from build123d import *

# Parameters (mm, degrees)
BASE_DEPTH                   = 12.7
BASE_DEPTH_BACK              = 12.7
SKETCH1_W                    = 43.18
SKETCH1_H                    = 108.204
ACTUATORPLANECUT_DEPTH       = 6.0325
CENTERSLOT_DEPTH             = 60.619162222
CENTERSLOT_DEPTH_BACK        = 60.619162222
SKETCH5_W                    = 25.654
SKETCH5_H                    = 19.05
SHAFTGUIDE_REACH             = 113.065
SKETCH2_R                    = 4.7625
CENTERSLOTFILLET_R           = 3.175
GEARBOXPIT_DEPTH             = 11.176
FRONTCUTAWAY_DEPTH           = 15.24
GEARBOXSLOTSH_DEPTH          = 2.286
TOGGLEASSEMHOLES_D           = 2.7051
TOGGLEASSEMHOLES_DEPTH       = 9.398
TOGGLEASSEMHOLES_TIP         = 0.81269403
GEARBOXMOUNTINGHOLES_D       = 2.7051
GEARBOXMOUNTINGHOLES_DEPTH   = 9.398
GEARBOXMOUNTINGHOLES_TIP     = 0.81269403
CAPMOUNTINGHOLES_D           = 3.6576
CAPMOUNTINGHOLES_CBORE_D     = 7.14502
CAPMOUNTINGHOLES_CBORE_DEPTH = 3.5052
ROLLMOTORSLOT_REACH          = 113.065


with BuildPart() as part:
    # Sketch1 → Base (new, two sides: drawn at the far end of the back side and taken through both)
    with BuildSketch(Plane(origin=(0, 0, 0), x_dir=(1, 0, 0), z_dir=(0, 1, 0)).offset(-BASE_DEPTH_BACK)):
        Rectangle(SKETCH1_W, SKETCH1_H)
    extrude(amount=BASE_DEPTH + BASE_DEPTH_BACK)

    # Sketch3 → ActuatorPlaneCut (cut)
    with BuildSketch(Plane(origin=(0, -12.7, 0), x_dir=(-1, 0, 0), z_dir=(0, -1, 0))):
        Polygon((10.922, -28.702), (16.256, -28.702), (21.59, -28.702), (21.59, -54.102), (-21.59, -54.102), (-21.59, -28.702), (-10.922, -28.702), (-10.922, -11.176), (10.922, -11.176), align=None)
    extrude(amount=-ACTUATORPLANECUT_DEPTH, mode=Mode.SUBTRACT)

    # Sketch5 → CenterSlot (cut, two sides: drawn at the far end of the back side and taken through both)
    with BuildSketch(Plane(origin=(0, 0, 0), x_dir=(1, 0, 0), z_dir=(0, 1, 0)).offset(-CENTERSLOT_DEPTH_BACK)):
        with Locations((0, 0.127)):
            Rectangle(SKETCH5_W, SKETCH5_H)
    extrude(amount=CENTERSLOT_DEPTH + CENTERSLOT_DEPTH_BACK, mode=Mode.SUBTRACT)

    # Sketch2 → ShaftGuide (cut, up to next)
    with BuildSketch(Plane(origin=(0, 0, -54.102), x_dir=(-1, 0, 0), z_dir=(0, 0, -1)), mode=Mode.PRIVATE) as shaftguide_sk1:
        with Locations((0, -12.7)):
            Circle(SKETCH2_R)
    shaftguide_tool1 = extrude(shaftguide_sk1.sketch, amount=-SHAFTGUIDE_REACH, mode=Mode.PRIVATE) & part.part
    add(shaftguide_tool1.solids().sort_by_distance((0, -12.7, -54.102))[0], mode=Mode.SUBTRACT)

    # CenterSlotFillet
    centerslotfillet_edges = [part.edges().sort_by_distance(p)[0] for p in [
        (-12.827, 0, -9.652),
        (-12.827, 0, 9.398),
        (12.827, 0, 9.398),
        (12.827, 0, -9.652),
    ]]
    fillet(centerslotfillet_edges, radius=CENTERSLOTFILLET_R)

    # Sketch40 → GearBoxPit (cut)
    with BuildSketch(Plane.XZ.offset(12.7)):
        with BuildLine():
            Line((10.922, 6.858), (-10.922, 6.858))
            Line((-10.922, 6.858), (-10.922, 25.527))
            ThreePointArc((-10.922, 25.527), (-9.99206403, 27.77206403), (-7.747, 28.702))
            Line((-7.747, 28.702), (7.747, 28.702))
            ThreePointArc((7.747, 28.702), (9.99206403, 27.77206403), (10.922, 25.527))
            Line((10.922, 25.527), (10.922, 6.858))
        make_face()
    extrude(amount=-GEARBOXPIT_DEPTH, mode=Mode.SUBTRACT)

    # Sketch60 → FrontCutaway (cut)
    with BuildSketch(Plane(origin=(0, 12.7, 0), x_dir=(1, 0, 0), z_dir=(0, 1, 0))):
        with BuildLine():
            Line((-12.827, 6.477), (12.827, 6.477))
            Line((12.827, 6.477), (12.827, 25.527))
            ThreePointArc((12.827, 25.527), (11.89706403, 27.77206403), (9.652, 28.702))
            Line((9.652, 28.702), (-9.652, 28.702))
            ThreePointArc((-9.652, 28.702), (-11.89706403, 27.77206403), (-12.827, 25.527))
            Line((-12.827, 25.527), (-12.827, 6.477))
        make_face()
    extrude(amount=-FRONTCUTAWAY_DEPTH, mode=Mode.SUBTRACT)

    # Sketch67 → GearBoxSlotsH (cut)
    with BuildSketch(Plane(origin=(0, -12.7, 0), x_dir=(-1, 0, 0), z_dir=(0, -1, 0))):
        with BuildLine():
            Line((-12.3825, -12.811125), (12.3825, -12.811125))
            ThreePointArc((12.3825, -12.811125), (12.779375, -13.208), (12.3825, -13.604875))
            Line((12.3825, -13.604875), (-12.3825, -13.604875))
            ThreePointArc((-12.3825, -13.604875), (-12.779375, -13.208), (-12.3825, -12.811125))
        make_face()
        with BuildLine():
            Line((-12.3825, -23.479125), (12.3825, -23.479125))
            ThreePointArc((12.3825, -23.479125), (12.779375, -23.876), (12.3825, -24.272875))
            Line((12.3825, -24.272875), (-12.3825, -24.272875))
            ThreePointArc((-12.3825, -24.272875), (-12.779375, -23.876), (-12.3825, -23.479125))
        make_face()
    extrude(amount=-GEARBOXSLOTSH_DEPTH, mode=Mode.SUBTRACT)

    # ToggleAssemHoles
    with Locations(Plane(origin=(0, -12.7, 0), x_dir=(-1, 0, 0), z_dir=(0, -1, 0))):
        with Locations((15.875, 22.352), (-15.875, 22.352)):
            Hole(TOGGLEASSEMHOLES_D / 2, depth=TOGGLEASSEMHOLES_DEPTH)
            with Locations((0, 0, -(TOGGLEASSEMHOLES_DEPTH + TOGGLEASSEMHOLES_TIP / 2))):  # 118° drill point
                Cone(0, TOGGLEASSEMHOLES_D / 2, TOGGLEASSEMHOLES_TIP, mode=Mode.SUBTRACT)

    # GearBoxMountingHoles
    with Locations(Plane(origin=(0, -12.7, 0), x_dir=(-1, 0, 0), z_dir=(0, -1, 0))):
        with Locations((-16.256, -18.542), (16.256, -18.542)):
            Hole(GEARBOXMOUNTINGHOLES_D / 2, depth=GEARBOXMOUNTINGHOLES_DEPTH)
            with Locations((0, 0, -(GEARBOXMOUNTINGHOLES_DEPTH + GEARBOXMOUNTINGHOLES_TIP / 2))):  # 118° drill point
                Cone(0, GEARBOXMOUNTINGHOLES_D / 2, GEARBOXMOUNTINGHOLES_TIP, mode=Mode.SUBTRACT)

    # CapMountingHoles (through all)
    with Locations(Plane(origin=(-0.837932951, 12.7, 8.633720573), x_dir=(-1, 0, 0), z_dir=(0, 1, 0))):
        with Locations((-13.537932951, 36.578279427), (11.862067049, 36.578279427)):
            CounterBoreHole(CAPMOUNTINGHOLES_D / 2, CAPMOUNTINGHOLES_CBORE_D / 2, CAPMOUNTINGHOLES_CBORE_DEPTH)

    # Sketch81 → RollMotorSlot (cut, up to next)
    with BuildSketch(Plane(origin=(0, 0, -54.102), x_dir=(-1, 0, 0), z_dir=(0, 0, -1)), mode=Mode.PRIVATE) as rollmotorslot_sk1:
        with BuildLine():
            Line((10.16, 12.7), (-10.16, 12.7))
            Line((-10.16, 12.7), (-10.16, 8.46582))
            ThreePointArc((-10.16, 8.46582), (-7.370192091, 1.730627909), (-0.635, -1.05918))
            Line((-0.635, -1.05918), (0.635, -1.05918))
            ThreePointArc((0.635, -1.05918), (7.370192091, 1.730627909), (10.16, 8.46582))
            Line((10.16, 8.46582), (10.16, 12.7))
        make_face()
    rollmotorslot_tool1 = extrude(rollmotorslot_sk1.sketch, amount=-ROLLMOTORSLOT_REACH, mode=Mode.PRIVATE) & part.part
    add(rollmotorslot_tool1.solids().sort_by_distance((0, 6.589347, -54.102))[0], mode=Mode.SUBTRACT)


solid = part.part
Geometry check sheet. Reference: the model listing, model coordinates, mm. A direction names the side the tool comes from. Round coordinates to 2 decimals unless told otherwise and drop trailing zeros. Loops run counter-clockwise (first coordinate to the right, second up) from the corner with the lowest first, then second, coordinate; pieces in that order, holes last. Notation, with made-up numbers: (-7.75, -10.75) - (44.25, -10.75) arc R31 cw to (44.25, 16.25) - close; hole circle Ø10 at (64.25, 89.5). An arc over 180 degrees is marked (long way). One line per question, with ' | ' between items. Start each with the question number.
1. Tool access check on faces 1 (the face through (-11.856, 1.153, 43.59)), 2 (the face through (15.259, -7.935, 17.628)), 3 (the face through (13, -12.7, -22)), 4 (the face through (13.474, 10.972, 41.724)), 5 (the face through (7.444, 1.805, -41.56)). Record the directions out of +Z, -Z, +X, -X, +Y, -Y that give a thin tool (end or side, any length) a straight path to the whole face; none if there is none.
2. Cross-section at B-B on x = 3. Record the cut outline in (y, z).
3. Cross-section at C-C on z = 38.5. Record the cut outline in (x, y).
4. Draft check along X on faces 6 (the face through (0, -3, -54.102)), 7 (the face through (10.16, 11, -42)). Enter one of: released by +X, released by -X, zero draft, split by the parting line, or undercut.
5. Scan lines: line 1 (X direction, y = -2.25, z = 45); line 2 (X direction, y = -0.25, z = 1.5); line 3 (X direction, y = -3, z = 23). Record each from-to range of solid material in increasing order. Write a range as [from, to].
6. Cross-section at A-A on z = -12.5. Record the cut outline in (x, y) (1 decimal).
7. Depth check by flat-ended pin: pin 1 (6 mm diameter, centred on x = -3, y = -10, fed in from +Z); pin 2 (3.5 mm diameter, centred on x = -12.7, z = 45.212, fed in from +Y); pin 3 (0.6 mm diameter, centred on x = 0, z = -46, fed in from +Y); pin 4 (2 mm diameter, centred on x = -11, z = 46, fed in from +Y). Enter the tip coordinate at first touch or a pass-through.
Taken from the geometry:
1) face 1: +Y, -Y | face 2: -Y | face 3: +Z, -Z, +X, -X, -Y | face 4: +Y | face 5: -Z, +Y
2) outline: (-9, -54.1) - (-0.76, -54.1) - (-0.76, -28.7) - (-2.54, -28.7) - (-2.54, -9.65) - (-9, -9.65) - close; (-6.67, 28.7) - (-1.52, 28.7) - (-1.52, 9.4) - (12.7, 9.4) - (12.7, 54.1) - (-6.67, 54.1) - close
3) outline: (-21.59, -6.67) - (21.59, -6.67) - (21.59, 12.7) - (-21.59, 12.7) - close
4) face 6: zero draft | face 7: undercut
5) line 1: [-21.59, -14.52], [-10.88, 10.88], [14.52, 21.59] | line 2: [-21.59, -12.83], [12.83, 21.59] | line 3: [-21.59, -10.92], [10.92, 21.59]
6) outline: (-21.6, -12.7) - (-4.8, -12.7) arc R4.8 cw to (4.8, -12.7) - (21.6, -12.7) - (21.6, 12.7) - (12.8, 12.7) - (12.8, -2.5) - (-12.8, -2.5) - (-12.8, 12.7) - (-21.6, 12.7) - close
7) pin 1: z = -9.65 | pin 2: through | pin 3: y = -1.06 | pin 4: y = 9.19
